Geometry check sheet. Reference: drawing and pictorial views, mm from the part's lowest x, y, z. Coordinates: 2 decimals unless noted, no trailing zeros. Order: outer loops, then holes, each group sorted by start corner. A loop starts at its lowest first (then second) coordinate and runs counter-clockwise, first axis right, second up. Notation, with made-up numbers: (10, -29.5) -> (53, -29.5) arc R28 ccw to (53, 4.5) -> close; hole circle Ø11 at (33.25, 31). An arc over 180 degrees is marked (long way). Use CSV: the item, a comma, the result in double quotes. Start each with the question number.
1) Scan lines: line 1 along Z through (x, y) = (21.5, 0.1) (1 decimal); line 2 along X through (y, z) = (1, 3) (1 decimal); line 3 along Z through (x, y) = (15.5, 0.55). Record each from-to range of solid material in increasing order.
2) Sectioned sample at B-B on z = 11. Record the boundary of the cut face in (x, y) (1 decimal).
3) Go/stop test with flat-tipped pins: pin 1 (2 mm diameter, centred on x = 25.5, z = 16, fed in from -Y); pin 2 (1 mm diameter, centred on x = 22, y = 0.5, fed in from +Z); pin 3 (1 mm diameter, centred on x = 28, y = 0.5, fed in from -Z); pin 4 (0.6 mm diameter, centred on x = 1.5, y = 1, fed in from +Z). Record where each tip stops, or that it passes through.
4) Sectioned sample at A-A on z = 28. Record the boundary of the cut face in (x, y) (1 decimal).
5) Sectioned sample at C-C on x = 16.5. Record the boundary of the cut face in (y, z).
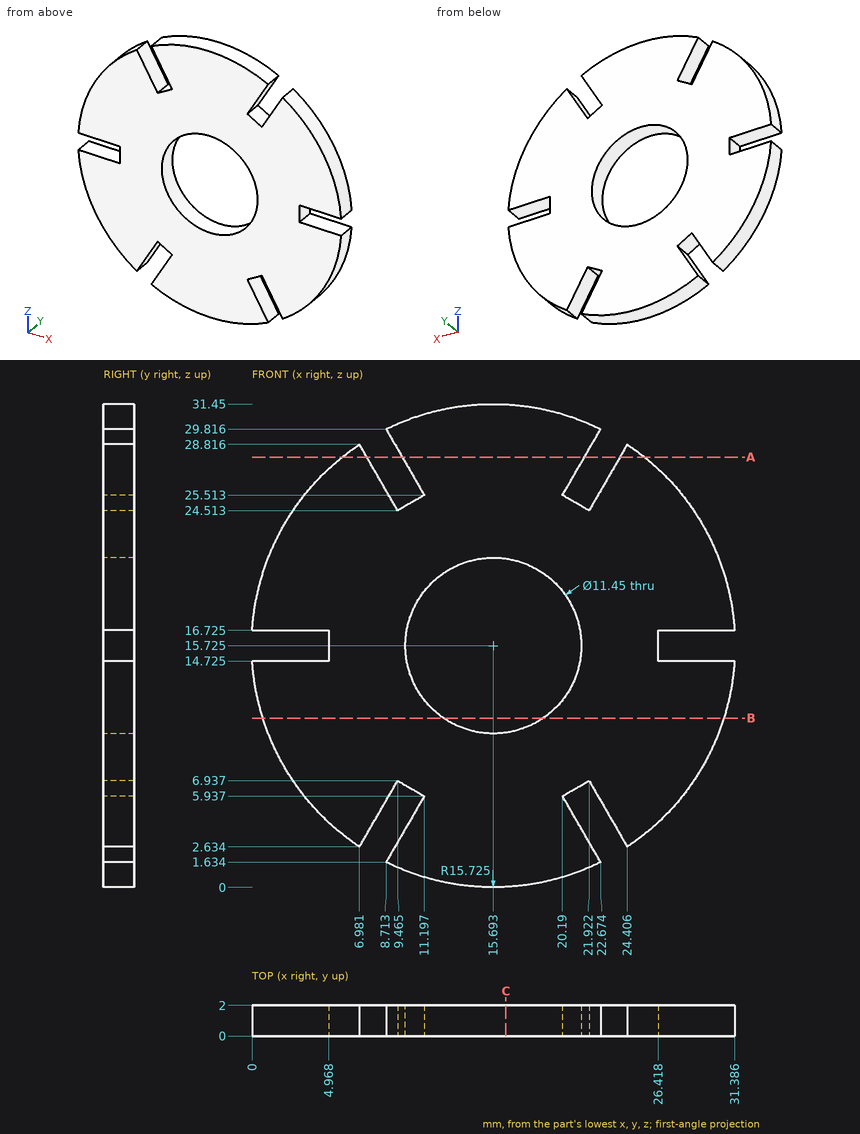
Answers follow:
1,line 1,"z = 1.1 to 3.7, 6.7 to 24.8, 27.8 to 30.3"
1,line 2,"x = 6.5 to 7.2, 9.5 to 21.9, 24.2 to 24.9"
1,line 3,"z = 0 to 10, 21.45 to 31.45"
2,outline,"(0.7, 0) -> (12.5, 0) -> (12.5, 2) -> (0.7, 2) -> close; (18.9, 0) -> (30.7, 0) -> (30.7, 2) -> (18.9, 2) -> close"
3,pin 1,"stops at y = 0"
3,pin 2,"stops at z = 30.34"
3,pin 3,"stops at z = 5.34"
3,pin 4,"stops at z = 23.09"
4,outline,"(5.9, 0) -> (7.5, 0) -> (7.5, 2) -> (5.9, 2) -> close; (9.8, 0) -> (21.6, 0) -> (21.6, 2) -> (9.8, 2) -> close; (23.9, 0) -> (25.5, 0) -> (25.5, 2) -> (23.9, 2) -> close"
5,outline,"(0, 0.02) -> (2, 0.02) -> (2, 10.06) -> (0, 10.06) -> close; (0, 21.39) -> (2, 21.39) -> (2, 31.43) -> (0, 31.43) -> close"
